```python
from build123d import *

# Parameters (mm, degrees)
SKETCH1_R           = 3
SKETCH1_R_2         = 1.5
BOSS_EXTRUDE1_DEPTH = 3


with BuildPart() as part:
    # Sketch1 → Boss-Extrude1 (new body)
    with BuildSketch(Plane(origin=(0, 0, 0), x_dir=(1, 0, 0), z_dir=(0, 1, 0))):
        Polygon((-42.867412192, 7), (-42.867412192, 10), (-39.867412192, 10), (-39.867412192, 13), (-9.867412192, 13), (-9.867412192, 10), (-6.867412192, 10), (-6.867412192, 7), (-9.867412192, 7), (-9.867412192, 0), (-6.867412192, 0), (-6.867412192, -3), (-9.867412192, -3), (-9.867412192, -6), (-39.867412192, -6), (-39.867412192, -3), (-42.867412192, -3), (-42.867412192, 0), (-39.867412192, 0), (-39.867412192, 7), align=None)
        with Locations((-24.867412192, 3.5)):
            Circle(SKETCH1_R, mode=Mode.SUBTRACT)
        with Locations((-34.867412192, 3.5)):
            Circle(SKETCH1_R_2, mode=Mode.SUBTRACT)
        with Locations((-14.867412192, 3.5)):
            Circle(SKETCH1_R_2, mode=Mode.SUBTRACT)
    extrude(amount=BOSS_EXTRUDE1_DEPTH)


solid = part.part
```
Can you work these out from the model? Positions are in its coordinate system, mm. A direction names the side the tool comes from. Coordinates: 2 decimals unless noted, no trailing zeros. Loops run counter-clockwise (first coordinate to the right, second up) from the corner with the lowest first, then second, coordinate; pieces in that order, holes last. Notation, with made-up numbers: M -4,-9 L 19,-9 A22 cw 19,14 Z; hole C -24.75,4 d7. An arc over 180 degrees is marked long. Put each result on its own line as item: value. Start each with the question number.
(1) Which directions (+Z, -Z, +X, -X, +Y, -Y) give clear straight access to the entire face, cutting with the end or side of a thin tool? Please do faces 1 (the face through (-8, 1, 3)), 2 (the face through (-41, 1, 3)), 3 (the face through (-39.867, 1, -3)), 4 (the face through (-9.867, 1, -12)).
(2) Imagine slicing it at D-D on z = -1.5. List the corners of the cut face in (x, y) for me, and give its area (3 significant figures).
(3) Will these pins go through, and if not, where does the flat tip stop? pin 1 Ø0.9 at (y, z) = (1.5, 5) entering from -X; pin 2 Ø2.5 at (x, z) = (-14.87, -3.5) entering from -Y; pin 3 Ø1.5 at (x, y) = (-9, 2) entering from +Z; pin 4 Ø1.5 at (y, z) = (1.5, -11.5) entering from +X.
(4) We'd pull the mould along Z, two halves only. Please class faces 5 (the face through (-33.437, 1.479, -3.951)), 6 (the face through (-8, 1, -10)), 7 (the face through (-42.867, 1, 2)): +Z half, -Z half, draft (parallel to the pull), parting line (faces both ways), or undercut.
(5) Imagine slicing it at A-A on z = -3.5. List the corners of the cut face in (x, y) for me.
(6) Imagine slicing it at C-C on y = 1.9. List the corners of the cut face in (x, z) for me, and give its area (3 significant figures).
(7) I need wall thicknesses on probe 1 along X at (y, z) = (1.55, -3.5); probe 2 along Z at (x, y) = (-41, 2.9); probe 3 along X at (y, z) = (2.5, -4.75). Which ranges of each line are inside material? Lowest first, please.
(8) Imagine slicing it at B-B on x = -26. List the corners of the cut face in (y, z) for me, and give its area (3 significant figures).
Worked answers:
1. face 1: +Z, +X, +Y, -Y
1. face 2: +Z, -X, +Y, -Y
1. face 3: -X, +Y, -Y
1. face 4: -Z, +X, +Y, -Y
2. outline: M -39.87,0 L -27.1,0 L -27.1,3 L -39.87,3 Z; M -22.63,0 L -9.87,0 L -9.87,3 L -22.63,3 Z
2. area: 76.6 mm2
3. pin 1: stops at x = -39.87
3. pin 2: passes through
3. pin 3: stops at z = 3
3. pin 4: stops at x = -9.87
4. face 5: undercut
4. face 6: -Z half
4. face 7: draft
5. outline: M -39.87,0 L -36.37,0 L -36.37,3 L -39.87,3 Z; M -33.37,0 L -27.87,0 L -27.87,3 L -33.37,3 Z; M -21.87,0 L -16.37,0 L -16.37,3 L -21.87,3 Z; M -13.37,0 L -9.87,0 L -9.87,3 L -13.37,3 Z
6. outline: M -42.87,-10 L -39.87,-10 L -39.87,-13 L -9.87,-13 L -9.87,-10 L -6.87,-10 L -6.87,-7 L -9.87,-7 L -9.87,0 L -6.87,0 L -6.87,3 L -9.87,3 L -9.87,6 L -39.87,6 L -39.87,3 L -42.87,3 L -42.87,0 L -39.87,0 L -39.87,-7 L -42.87,-7 Z; hole C -34.87,-3.5 d3; hole C -24.87,-3.5 d6; hole C -14.87,-3.5 d3
6. area: 564 mm2
7. probe 1: x = -39.87 to -36.37, -33.37 to -27.87, -21.87 to -16.37, -13.37 to -9.87
7. probe 2: z = -10 to -7, 0 to 3
7. probe 3: x = -39.87 to -35.7, -34.04 to -27.59, -22.14 to -15.7, -14.04 to -9.87
8. outline: M 0,-13 L 3,-13 L 3,-6.28 L 0,-6.28 Z; M 0,-0.72 L 3,-0.72 L 3,6 L 0,6 Z
8. area: 40.3 mm2
